Source: CAD feature listing. Evaluate the final solid. Frame: model axes, mm. Coordinates: 2 decimals unless noted, no trailing zeros. Loops run counter-clockwise (first coordinate to the right, second up) from the corner with the lowest first, then second, coordinate; pieces in that order, holes last. Notation, with made-up numbers: M -33,2 L 12,2 A24 ccw 12,41 Z; hole C 33,71 d5. An arc over 180 degrees is marked long. One line per question, with ' | ' between items. Start each with the question number.
1. Section query B-B, the plane x = 18. Output: boundary loops of the cut face in (y, z).
2. Section query A-A, the plane z = 0. Output: boundary loops of the cut face in (x, y).
3. Pin query (flat end, axial travel): P1, Ø2.5, axis at x = 18, z = 0, coming from the +Y side. Return the tip coordinate at first contact, or that it passes through.
4. Mould query, pull axis Z, two halves, no side actions, for faces 1 (the cylindrical face through (19.31, 6.41, 1)), 2 (the flat face through (37.5, 6, 0)), 3 (the cylindrical face through (-19.574, 6.409, -0.496)), 4 (the cylindrical face through (36.748, 6.591, -11.787)). Classes: pulls with the +Z half, pulls with the -Z half, needs draft (parallel to the pull), parting line crosses it, or undercut.
5. Ray query, probe 1 along Z at (x, y) = (-18, 6.5); probe 2 along X at (y, z) = (9, -0.25); probe 3 along X at (y, z) = (1.25, -10.5). Return the intervals inside material, ascending.
```python
from build123d import *

# Parameters (mm, degrees)
SKETCH1_W                   = 75
SKETCH1_H                   = 25
BOSS_EXTRUDE1_DEPTH         = 13
TAP_DRILL_FOR_M4X0_7_TAP1_D = 3.3
FILLET1_R                   = 2.5


with BuildPart() as part:
    # Sketch1 → Boss-Extrude1 (new body)
    with BuildSketch(Plane(origin=(0, 0, 0), x_dir=(1, 0, 0), z_dir=(0, 1, 0))):
        Rectangle(SKETCH1_W, SKETCH1_H)
    extrude(amount=BOSS_EXTRUDE1_DEPTH)

    # Tap Drill for M4x0.7 Tap1 (through all)
    with Locations(Plane(origin=(0, 13, 0), x_dir=(1, 0, 0), z_dir=(0, 1, 0))):
        with Locations((-18, 0), (18, 0)):
            Hole(TAP_DRILL_FOR_M4X0_7_TAP1_D / 2)

    # Fillet1
    fillet1_edges = [part.edges().sort_by_distance(p)[0] for p in [
        (37.5, 6.5, 12.5),
        (-37.5, 6.5, 12.5),
        (-37.5, 6.5, -12.5),
        (37.5, 6.5, -12.5),
    ]]
    fillet(fillet1_edges, radius=FILLET1_R)


solid = part.part
```
Taken from the geometry:
1) outline: M 0,-12.5 L 13,-12.5 L 13,-1.65 L 0,-1.65 Z; M 0,1.65 L 13,1.65 L 13,12.5 L 0,12.5 Z
2) outline: M -37.5,0 L -19.65,0 L -19.65,13 L -37.5,13 Z; M -16.35,0 L 16.35,0 L 16.35,13 L -16.35,13 Z; M 19.65,0 L 37.5,0 L 37.5,13 L 19.65,13 Z
3) P1: through
4) face 1: undercut | face 2: needs draft | face 3: undercut | face 4: pulls with the -Z half
5) probe 1: -12.5 to -1.65, 1.65 to 12.5 | probe 2: -37.5 to -19.63, -16.37 to 16.37, 19.63 to 37.5 | probe 3: -37.45 to 37.45
